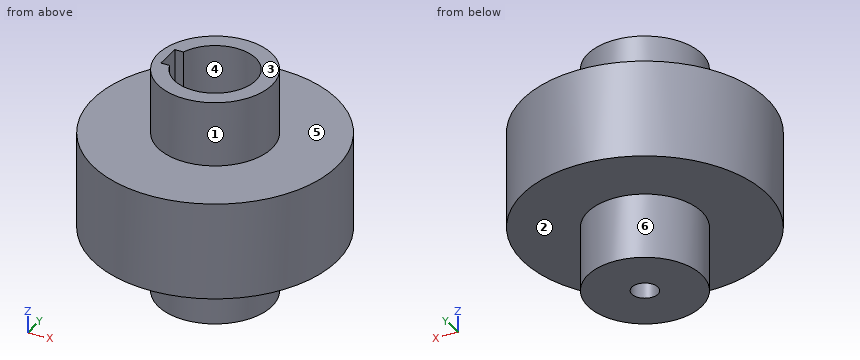
Autodesk Inventor part; units mm, degrees
ref_plane "YZ Plane" through (0, 0, 0) normal (1, 0, 0) x (0, 1, 0)
ref_plane "XZ Plane" through (0, 0, 0) normal (0, 1, 0) x (-1, 0, 0)
ref_plane "XY Plane" through (0, 0, 0) normal (0, 0, 1) x (1, 0, 0)
sketch "Sketch1" plane through (0, 0, 0) normal (0, 0, 1) x (1, 0, 0)
  circle A0 centre (0, 0) radius 37.5
  dimension "d0" = 75
extrude "Extrusion1" add sketch "Sketch1" along normal mid plane 30
sketch "Sketch2" plane through (0, 0, 15) normal (0, 0, 1) x (1, 0, 0)
  circle A0 centre (0, 0) radius 17.5
  circle A1 centre (0, 0) radius 12.5
  dimension "d3" = 35
  dimension "d4" = 25
extrude "Extrusion2" add sketch "Sketch2" along normal blind 20
sketch "Sketch3" plane through (0, 0, 35) normal (0, 0, 1) x (1, 0, 0)
  line L0 (-10.5, -4) -> (-14.5, -4)
  line L1 (-14.5, -4) -> (-14.5, 4)
  line L2 (-14.5, 4) -> (-10.5, 4)
  line L3 (-10.5, 4) -> (-10.5, -4)
  circle A0 centre (0, 0) radius 12.5
  line L4 (-10.5, -4) -> (-14.5, 4) construction
  line L5 (-14.5, -4) -> (-10.5, 4) construction
  point P0 (-12.5, 0)
  point P1 (-11.8427, -4)
  point P2 (-11.8427, 4)
  dimension "d7" = 4
  dimension "d8" = 8
extrude "Extrusion3" cut sketch "Sketch3" against normal blind 20 contours L0 L1 L2 A0
sketch "Sketch4" plane through (0, 0, -15) normal (0, 0, -1) x (-1, 0, 0)
  circle A0 centre (0, 0) radius 17.5
  circle A1 centre (0, 0) radius 4
  dimension "d11" = 8
extrude "Extrusion4" add sketch "Sketch4" along normal blind 20
sketch "Sketch5" plane through (0, 0, -35) normal (0, 0, -1) x (-1, 0, 0)
  point P0 (0, 0)
properties part number "pump and e-motor coupling"
Verification items for the finished model (mm, model axes). Face numbers are marked on the shaded views. A direction names the side the tool comes from. Give positions to 0.01 mm unless a question says otherwise; leave off trailing zeros. Loops run counter-clockwise (first coordinate to the right, second up) from the corner with the lowest first, then second, coordinate; pieces in that order, holes last.
1. Cross-section at B-B on y = -14.5. Record the cut outline in (x, z).
Derived:
outline: (-34.58, -15) - (-9.8, -15) - (-9.8, -35) - (9.8, -35) - (9.8, -15) - (34.58, -15) - (34.58, 15) - (9.8, 15) - (9.8, 35) - (-9.8, 35) - (-9.8, 15) - (-34.58, 15) - close
2. Tool access check on the marked faces 1, 2 and 3. Record the directions out of +Z, -Z, +X, -X, +Y, -Y that give a thin tool (end or side, any length) a straight path to the whole face; none if there is none.
Derived:
face 1: +Z
face 2: -Z
face 3: +Z, +X, -X, +Y, -Y
3. Go/stop test with flat-tipped pins: P1, Ø12.5, axis at x = 2.5, y = 1.5, coming from the +Z side; P2, Ø2, axis at y = -6, z = 13, coming from the +X side; P3, Ø6, axis at y = -22.5, z = -20, coming from the +X side; P4, Ø6, axis at x = -0.5, z = -18.5, coming from the -Y side. Record where each tip stops, or that it passes through.
Derived:
P1: stops at z = 15
P2: stops at x = 37.17
P3: passes through
P4: stops at y = -17.5
4. Cross-section at A-A on z = -19. Record the cut outline in (x, y), and give its area (3 significant figures).
Derived:
outline: circle Ø35 at (0, 0); hole circle Ø8 at (0, 0)
area: 912 mm2
5. Cross-section at C-C on x = 0. Record the cut outline in (y, z).
Derived:
outline: (-37.5, -15) - (-17.5, -15) - (-17.5, -35) - (-4, -35) - (-4, -15) - (4, -15) - (4, -35) - (17.5, -35) - (17.5, -15) - (37.5, -15) - (37.5, 15) - (17.5, 15) - (17.5, 35) - (12.5, 35) - (12.5, 15) - (-12.5, 15) - (-12.5, 35) - (-17.5, 35) - (-17.5, 15) - (-37.5, 15) - close
6. Material ranges on probe 1 along Y at (x, z) = (0, 24); probe 2 along Y at (x, z) = (0, -26.25); probe 3 along Z at (x, y) = (-1.5, -22.5), recorded low to high.
Derived:
probe 1: y = -17.5 to -12.5, 12.5 to 17.5
probe 2: y = -17.5 to -4, 4 to 17.5
probe 3: z = -15 to 15
7. Release check for a two-part mould opening along X. For the marked faces 4, 5 and 6 record: +X half, -X half, draft (parallel to the pull), parting line (faces both ways), or undercut.
Derived:
face 4: undercut
face 5: draft
face 6: parting line
8. Cross-section at D-D on y = 0. Record the cut outline in (x, z), and give its area (3 significant figures).
Derived:
outline: (-37.5, -15) - (-17.5, -15) - (-17.5, -35) - (-4, -35) - (-4, -15) - (4, -15) - (4, -35) - (17.5, -35) - (17.5, -15) - (37.5, -15) - (37.5, 15) - (17.5, 15) - (17.5, 35) - (12.5, 35) - (12.5, 15) - (-14.5, 15) - (-14.5, 35) - (-17.5, 35) - (-17.5, 15) - (-37.5, 15) - close
area: 2,950 mm2
